```python
from build123d import *

# Parameters (mm, degrees)
F0_W    = 76.2
F0_H    = 22.225
F2_SIZE = 5.08
F3_T    = -2.54


with BuildPart() as f1:
    # F0 (on Front) → F1 (revolve)
    with BuildSketch(Plane.XZ):
        with Locations((0, 50.8)):
            Rectangle(F0_W, F0_H)
    revolve(axis=Axis((-6.255699, 0, 0), (1, 0, 0)))

    # F2
    f2_edges = [f1.edges().sort_by_distance(p)[0] for p in [
        (-38.1, 0, -61.9125),
    ]]
    chamfer(f2_edges, length=F2_SIZE)

    # F3
    f3_openings = [f1.faces().sort_by_distance(p)[0] for p in [
        (38.1, 0, -41.43865),
    ]]
    offset(amount=F3_T, openings=f3_openings)


solid = f1.part
```
Build history of the part. All positions in model axes, mm. A direction names the side the tool comes from. Round coordinates to 2 decimals unless told otherwise and drop trailing zeros. Write each loop counter-clockwise with the first axis right and the second up, starting at its lowest first coordinate (ties: lowest second). Pieces come first, ordered by that corner, then holes.
1) 3-axis set-ups, long thin cutter, end or side, ignore diameter. For faces 1 (the cylindrical face through (0.533, -11.921, 37.855)), 2 (the cylindrical face through (3.56, -17.83, 56.63)): which of +Z, -Z, +X, -X, +Y, -Y reach the whole face in a straight line?
2) Band-saw the part on A-A, the plane z = 0. List the corners of the cut face in (x, y).
3) Mould opens along Z. For faces 3 (the cylindrical face through (3.04, 60.44, -13.42)), 4 (the flat face through (-38.1, -39, -12)), 5 (the cylindrical face through (1.79, 37.46, 19.49)) say: +Z half, -Z half, draft (parallel to the pull), parting line (faces both ways), or undercut.
4) Band-saw the part on C-C, the plane x = 7. List the corners of the cut face in (y, z) (1 decimal).
5) Pin check, flat tips, straight feed: pin 1 (3 mm diameter, centred on x = -8, y = 35.5, fed in from -Z); pin 2 (6 mm diameter, centred on x = -9, z = -41.5, fed in from -Y); pin 3 (3 mm diameter, centred on x = 10.5, y = -7.5, fed in from -Z). Stop position of each tip, or through.
6) Drill centre lines: probe 1 along Z at (x, y) = (-6, 0); probe 2 along Z at (x, y) = (-19, 10). Where is each one in solid material? Low to high.
Ans:
1. face 1: +X, -X
1. face 2: +X
2. outline: (-38.1, -56.83) - (-33.02, -61.91) - (38.1, -61.91) - (38.1, -59.37) - (-31.97, -59.37) - (-35.56, -55.78) - (-35.56, -42.23) - (38.1, -42.23) - (38.1, -39.69) - (-38.1, -39.69) - close; (-38.1, 39.69) - (38.1, 39.69) - (38.1, 42.23) - (-35.56, 42.23) - (-35.56, 55.78) - (-31.97, 59.37) - (38.1, 59.37) - (38.1, 61.91) - (-33.02, 61.91) - (-38.1, 56.83) - close
3. face 3: parting line
3. face 4: draft
3. face 5: undercut
4. outline: circle Ø123.8 at (0, 0); circle Ø84.5 at (0, 0); hole circle Ø118.7 at (0, 0); hole circle Ø79.4 at (0, 0)
5. pin 1: stops at z = -51.74
5. pin 2: stops at y = -48.49
5. pin 3: stops at z = -61.62
6. probe 1: z = -61.91 to -59.37, -42.23 to -39.69, 39.69 to 42.23, 59.37 to 61.91
6. probe 2: z = -61.1 to -58.52, -41.03 to -38.41, 38.41 to 41.03, 58.52 to 61.1
